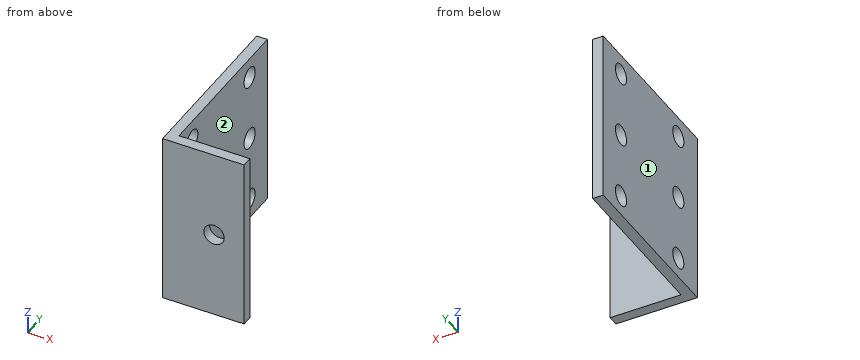
from build123d import *

# Parameters (mm, degrees)
SKETCH2_W                   = 25.4
SKETCH2_H                   = 54.102
BOSS_EXTRUDE1_DEPTH         = 3.302
SKETCH3_W                   = 3.302
SKETCH3_H                   = 54.102
BOSS_EXTRUDE2_DEPTH         = 50.546
F_1_4_0_25_DIAMETER_HOLE1_D = 6.35
F_1_4_0_25_DIAMETER_HOLE3_D = 6.35


with BuildPart() as part:
    # Sketch2 → Boss-Extrude1 (new body)
    with BuildSketch(Plane(origin=(0, 0, 0), x_dir=(1, 0, 0), z_dir=(0, 1, 0))):
        Rectangle(SKETCH2_W, SKETCH2_H)
    extrude(amount=BOSS_EXTRUDE1_DEPTH)

    # Sketch3 → Boss-Extrude2 (add)
    with BuildSketch(Plane(origin=(0, 3.302, 0), x_dir=(1, 0, 0), z_dir=(0, 1, 0))):
        with Locations((-11.049, 0)):
            Rectangle(SKETCH3_W, SKETCH3_H)
    extrude(amount=BOSS_EXTRUDE2_DEPTH)

    # 1/4 (0.25) Diameter Hole1 (through all)
    with Locations(Plane(origin=(-9.398, 0, 0), x_dir=(0, 0, -1), z_dir=(1, 0, 0))):
        with Locations((-20.701, 43.685729795), (0, 43.685729795), (20.701, 43.685729795), (20.701, 10.909480531), (0, 10.909480531), (-20.701, 10.909480531)):
            Hole(F_1_4_0_25_DIAMETER_HOLE1_D / 2)

    # 1/4 (0.25) Diameter Hole3 (through all)
    with Locations(Plane(origin=(0, 3.302, 0), x_dir=(1, 0, 0), z_dir=(0, 1, 0))):
        with Locations((3.302, 0)):
            Hole(F_1_4_0_25_DIAMETER_HOLE3_D / 2)


solid = part.part
Verification items for the finished model (mm, model axes). Face numbers are marked on the shaded views. A direction names the side the tool comes from. Coordinates: 2 decimals unless noted, no trailing zeros. Order: outer loops, then holes, each group sorted by start corner. A loop starts at its lowest first (then second) coordinate and runs counter-clockwise, first axis right, second up. Notation, with made-up numbers: M 34,-25 L 55,-25 A19 cw 55,-3 Z; hole C -2.75,74 d8. An arc over 180 degrees is marked long. One line per item, written item: value. Start each with the question number.
Item 1: Access from +Z, -Z, +X, -X, +Y, -Y to the whole of each face (thin tool, end or side, straight path). Record for the marked faces 1 and 2.
Item 2: Sectioned sample at B-B (x = 5.5). Enter the section's corners in (y, z).
Item 3: Scan lines: probe 1 along Y at (x, z) = (-11.75, 0); probe 2 along X at (y, z) = (19.5, 18.5); probe 3 along Y at (x, z) = (9.5, 23). Record each from-to range of solid material in increasing order.
Item 4: Gauge pin test, flat ends, axial feed: pin 1 (6 mm diameter, centred on y = 25.5, z = 1, fed in from +X); pin 2 (12 mm diameter, centred on x = 4.5, z = 15, fed in from +Y); pin 3 (5 mm diameter, centred on y = 43.69, z = -20.7, fed in from +X). Record the tip position at first contact, or that the pin passes through.
Item 5: Sectioned sample at C-C (y = 44.5). Enter the section's corners in (x, z).
Item 6: Sectioned sample at A-A (z = 0). Enter the section's corners in (x, y), then the cut area to 3 significant figures.
Item 7: Sectioned sample at D-D (z = 9). Enter the section's corners in (x, y).
Conclusion:
1. face 1: +Z, -Z, -X, +Y, -Y
1. face 2: +Z, -Z, +X, +Y
2. outline: M 0,-27.05 L 3.3,-27.05 L 3.3,-2.29 L 0,-2.29 Z; M 0,2.29 L 3.3,2.29 L 3.3,27.05 L 0,27.05 Z
3. probe 1: y = 0 to 7.73, 14.08 to 40.51, 46.86 to 53.85
3. probe 2: x = -12.7 to -9.4
3. probe 3: y = 0 to 3.3
4. pin 1: stops at x = -9.4
4. pin 2: stops at y = 3.3
4. pin 3: passes through
5. outline: M -12.7,-27.05 L -9.4,-27.05 L -9.4,-23.77 L -12.7,-23.77 Z; M -12.7,-17.63 L -9.4,-17.63 L -9.4,-3.07 L -12.7,-3.07 Z; M -12.7,3.07 L -9.4,3.07 L -9.4,17.63 L -12.7,17.63 Z; M -12.7,23.77 L -9.4,23.77 L -9.4,27.05 L -12.7,27.05 Z
6. outline: M -12.7,0 L 0.13,0 L 0.13,3.3 L -9.4,3.3 L -9.4,7.73 L -12.7,7.73 Z; M -12.7,14.08 L -9.4,14.08 L -9.4,40.51 L -12.7,40.51 Z; M -12.7,46.86 L -9.4,46.86 L -9.4,53.85 L -12.7,53.85 Z; M 6.48,0 L 12.7,0 L 12.7,3.3 L 6.48,3.3 Z
6. area: 188 mm^2
7. outline: M -12.7,0 L 12.7,0 L 12.7,3.3 L -9.4,3.3 L -9.4,53.85 L -12.7,53.85 Z
